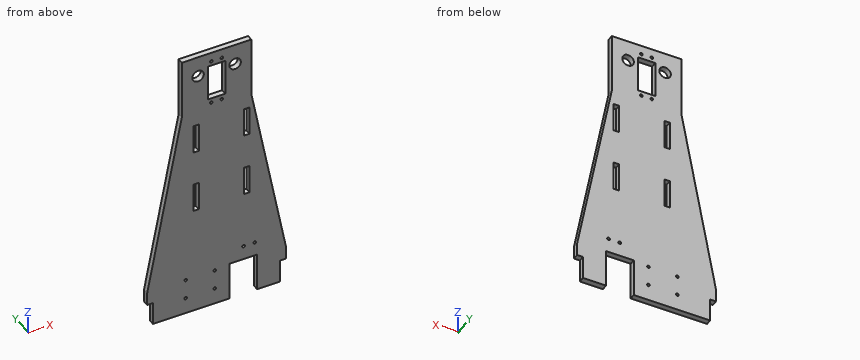
from build123d import *

# Parameters (mm, degrees)
SKETCH1_R           = 1.55
BOSS_EXTRUDE1_DEPTH = 6.35
SKETCH4_R           = 6.35
SKETCH4_W           = 6.35
SKETCH4_H           = 25.4
CUT_EXTRUDE2_DEPTH  = 250.304006214
SKETCH5_R           = 1.5
SKETCH5_W           = 19.05
SKETCH5_H           = 39.878
CUT_EXTRUDE3_DEPTH  = 250.304006214
SKETCH9_W           = 6.077459071
SKETCH9_H           = 31.906291655
SKETCH9_H_2         = 31.906291656
CUT_EXTRUDE4_DEPTH  = 37.338


with BuildPart() as part:
    # Sketch1 → Boss-Extrude1 (new body)
    with BuildSketch(Plane(origin=(0, 0, 0), x_dir=(1, 0, 0), z_dir=(0, 1, 0))):
        Polygon((-90.17, 72.46073058), (-90.17, 32.83673058), (-52.07, -166.371605632), (-52.07, -232.33926942), (24.13, -232.33926942), (24.13, -166.371605632), (62.23, 32.83673058), (62.23, 72.46073058), (30.48, 72.46073058), (30.48, 30.55073058), (0, 30.55073058), (0, 72.46073058), align=None)
        with Locations(Location((15.621, 14.819934213, 0), (0, 0, 270))):
            Circle(SKETCH1_R, mode=Mode.SUBTRACT)
        with Locations(Location((27.813, 14.819934213, 0), (0, 0, 270))):
            Circle(SKETCH1_R, mode=Mode.SUBTRACT)
    extrude(amount=BOSS_EXTRUDE1_DEPTH)

    # Sketch4 → Cut-Extrude2 (cut, through all)
    with BuildSketch(Plane(origin=(0, 6.35, 0), x_dir=(1, 0, 0), z_dir=(0, 1, 0))):
        with Locations(Location((-34.29, -209.515437526, 0), (0, 0, 270))):
            Circle(SKETCH4_R)
        with Locations(Location((6.35, -209.515437526, 0), (0, 0, 90))):
            Circle(SKETCH4_R)
        with Locations((59.055, 59.76073058)):
            Rectangle(SKETCH4_W, SKETCH4_H)
        with Locations((-86.995, 59.76073058)):
            Rectangle(SKETCH4_W, SKETCH4_H)
    extrude(amount=-CUT_EXTRUDE2_DEPTH, mode=Mode.SUBTRACT)

    # Sketch5 → Cut-Extrude3 (cut, through all)
    with BuildSketch(Plane(origin=(0, 6.35, 0), x_dir=(1, 0, 0), z_dir=(0, 1, 0))):
        with Locations(Location((-19.685, -222.17926942, 0), (0, 0, 270))):
            Circle(SKETCH5_R)
        with Locations(Location((-8.255, -222.17926942, 0), (0, 0, 270))):
            Circle(SKETCH5_R)
        with Locations(Location((-19.685, -172.14126942, 0), (0, 0, 270))):
            Circle(SKETCH5_R)
        with Locations(Location((-8.255, -172.14126942, 0), (0, 0, 270))):
            Circle(SKETCH5_R)
        with Locations(Location((-16.002, 54.42673058, 0), (0, 0, 270))):
            Circle(SKETCH5_R)
        with Locations(Location((-47.752, 54.42673058, 0), (0, 0, 270))):
            Circle(SKETCH5_R)
        with Locations(Location((-47.752, 32.58273058, 0), (0, 0, 270))):
            Circle(SKETCH5_R)
        with Locations(Location((-16.002, 32.58273058, 0), (0, 0, 270))):
            Circle(SKETCH5_R)
        with Locations((-13.97, -197.16026942)):
            Rectangle(SKETCH5_W, SKETCH5_H)
    extrude(amount=-CUT_EXTRUDE3_DEPTH, mode=Mode.SUBTRACT)

    # Sketch9 → Cut-Extrude4 (cut)
    with BuildSketch(Plane(origin=(0, 0, 0), x_dir=(1, 0, 0), z_dir=(0, 1, 0))):
        with Locations((19.088272024, -134.811490569)):
            Rectangle(SKETCH9_W, SKETCH9_H)
        with Locations((19.088272024, -63.999553047)):
            Rectangle(SKETCH9_W, SKETCH9_H_2)
        with Locations((-36.522018281, -134.811490569)):
            Rectangle(SKETCH9_W, SKETCH9_H)
        with Locations((-36.522018281, -63.999553047)):
            Rectangle(SKETCH9_W, SKETCH9_H_2)
    extrude(amount=CUT_EXTRUDE4_DEPTH, mode=Mode.SUBTRACT)


solid = part.part
The model under review builds one solid part; all positions refer to its coordinate system, in mm. Give positions to 0.01 mm unless a question says otherwise; leave off trailing zeros. Loops run counter-clockwise (first coordinate to the right, second up) from the corner with the lowest first, then second, coordinate; pieces in that order, holes last. Notation, with made-up numbers: (51, -32) -> (103, -32) arc R23 ccw to (103, -17) -> close; hole circle Ø5 at (38.5, 45). An arc over 180 degrees is marked (long way). Answer as a JSON object with one key per item and string values. Group by question number.
Q1. Take a section at B-B (z = -20.5). Write out the cut boundary in (x, y), plus the area to 3 significant figures.
Q2. Take a section at C-C (y = 5). State how many separate pieces and enclosed holes the cut face has, plus the area to 3 significant figures.
Q3. Wall thickness on line 1 along Z through (x, y) = (-47.5, 1.5); line 2 along Z through (x, y) = (-8.5, 4.5); line 3 along Z through (x, y) = (-13, 4.75): over which ranges is each line inside the solid? List them lowest first.
Q4. Take a section at A-A (x = 6.35). Write out the cut boundary in (y, z).
Q5. Insertion check: pin 1 (1.5 mm diameter, centred on y = 4.5, z = 118, fed in from +X); pin 2 (1.9 mm diameter, centred on y = 3, z = 58, fed in from -X); pin 3 (3 mm diameter, centred on y = 4, z = 70, fed in from +X). Each pin has a flat end and moves straight along its axis. Give the tip position at first contact, or say it passes through.
Q6. Take a section at D-D (x = 38). Write out the cut boundary in (y, z).
Answer below:
{
 "1": {"outline": "(-87.81, 0) -> (59.87, 0) -> (59.87, 6.35) -> (-87.81, 6.35) -> close", "area": "938 mm2"},
 "2": {"separate pieces": "1", "enclosed holes": "17", "area": "30,400 mm2"},
 "3": {"line 1": "z = -72.46 to -55.91, -52.95 to -34.06, -31.1 to 232.34", "line 2": "z = -72.46 to 170.66, 173.62 to 177.22, 217.1 to 220.7, 223.66 to 232.34", "line 3": "z = -72.46 to 177.22, 217.1 to 232.34"},
 "4": {"outline": "(0, -30.55) -> (6.35, -30.55) -> (6.35, 203.17) -> (0, 203.17) -> close; (0, 215.87) -> (6.35, 215.87) -> (6.35, 232.34) -> (0, 232.34) -> close"},
 "5": {"pin 1": "stops at x = 33.52", "pin 2": "stops at x = -72.98", "pin 3": "stops at x = 42.85"},
 "6": {"outline": "(0, -72.46) -> (6.35, -72.46) -> (6.35, 93.85) -> (0, 93.85) -> close"}
}
